Autodesk Inventor part; units mm, degrees
ref_plane "YZ Plane" through (0, 0, 0) normal (1, 0, 0) x (0, 1, 0)
ref_plane "XZ Plane" through (0, 0, 0) normal (0, 1, 0) x (-1, 0, 0)
ref_plane "XY Plane" through (0, 0, 0) normal (0, 0, 1) x (1, 0, 0)
sketch "Sketch1" plane through (0, 0, 0) normal (0, 1, 0) x (-1, 0, 0)
  line L0 (52.5, 30) -> (-52.5, 30)
  line L1 (-52.5, 30) -> (-52.5, -30)
  line L2 (-52.5, -30) -> (52.5, -30)
  line L3 (52.5, -30) -> (52.5, 30)
  line L4 (52.5, 0) -> (-52.5, 0) construction
  circle A0 centre (-42.5, 0) radius 1.5
  circle A1 centre (-0.5, 0) radius 1.5
  line L5 (-47.5, 25) -> (47.5, 25) construction
  line L6 (47.5, 25) -> (47.5, -25) construction
  line L7 (47.5, -25) -> (-47.5, -25) construction
  line L8 (-47.5, -25) -> (-47.5, 25) construction
  circle A2 centre (47.5, 25) radius 1.5
  circle A3 centre (47.5, -25) radius 1.5
  circle A4 centre (-47.5, 25) radius 1.5
  circle A5 centre (-47.5, -25) radius 1.5
  line L9 (47.5, 0) -> (34.5096, -7.5)
  line L10 (34.5096, -7.5) -> (34.5096, 7.5)
  line L11 (34.5096, 7.5) -> (47.5, 0)
  circle A6 centre (9.5, -13) radius 1
  circle A7 centre (9.5, 13) radius 1
  line L12 (9.5, -30) -> (9.5, 30) construction
  point P0 (0, 0)
  point P1 (0, 0)
  point P2 (38.8397, 0)
  dimension "d0" = 105
  dimension "d1" = 60
  dimension "d2" = 3
  dimension "d3" = 3
  dimension "d4" = 42
  dimension "d5" = 5
  dimension "d6" = 3
  dimension "d7" = 3
  dimension "d8" = 3
  dimension "d9" = 3
  dimension "d10" = 15
  dimension "d11" = 10
  dimension "d17" = 2
  dimension "d18" = 2
  dimension "d19" = 26
  dimension "d20" = 10
extrude "Extrusion1" add sketch "Sketch1" along normal blind 3
chamfer "Chamfer1" distance 2 angle 45 3 edges at (-41.0048, 3, -3.75) (-41.0048, 3, 3.75) (-34.5096, 3, 0)
properties part number "Front back" material "Iron, Gray"
Check sheet for the modelled part. Datum: model origin and axes. Units: mm. A direction names the side the tool comes from. Round coordinates to 2 decimals unless told otherwise and drop trailing zeros. Write each loop counter-clockwise with the first axis right and the second up, starting at its lowest first coordinate (ties: lowest second). Pieces come first, ordered by that corner, then holes. Notation, with made-up numbers: (20.25, 57.25) -> (63.25, 57.25) arc R20 cw to (63.25, 74.25) -> close; hole circle Ø3 at (-39.5, -8.5). An arc over 180 degrees is marked (long way). One line per question, with ' | ' between items. Start each with the question number.
1. Sectioned sample at A-A, the plane x = 47.5. Record the cut outline in (y, z), then the cut area to 3 significant figures.
2. Sectioned sample at B-B, the plane z = 13. Record the cut outline in (x, y).
3. Depth check by flat-ended pin: pin 1 (4 mm diameter, centred on x = -47.5, z = -25, fed in from -Y). Enter the tip coordinate at first touch or a pass-through.
4. Scan lines: line 1 along Z through (x, y) = (47.5, 1.3); line 2 along X through (y, z) = (1.25, 24.5); line 3 along Z through (x, y) = (-47.5, 1.5). Record each from-to range of solid material in increasing order. Write a range as from..to.
5. Set-up check for faces 5 (the face through (52.5, 1, 0)), 6 (the face through (-41.38, 2.01, -4.7)), 7 (the face through (-40.914, 0.493, 3.803)): record each of +Z, -Z, +X, -X, +Y, -Y from which the full face is reachable in a straight line by a thin tool's end or side.
6. Release check for a two-part mould opening along X. For faces 1 (the face through (44, 1, 0)), 2 (the face through (-52.5, 1, 0)), 3 (the face through (-46.39, 1.48, 23.99)), 4 (the face through (-1, 1, 30)) record: +X half, -X half, draft (parallel to the pull), parting line (faces both ways), or undercut.
7. Sectioned sample at C-C, the plane y = 2.45. Count the separate pieces of the cut face and the enclosed holes in it, then the cut area to 3 significant figures.
Taken from the geometry:
1) outline: (0, -30) -> (3, -30) -> (3, -26.5) -> (0, -26.5) -> close; (0, -23.5) -> (3, -23.5) -> (3, 23.5) -> (0, 23.5) -> close; (0, 26.5) -> (3, 26.5) -> (3, 30) -> (0, 30) -> close | area: 162 mm^2
2) outline: (-52.5, 0) -> (-10.5, 0) -> (-10.5, 3) -> (-52.5, 3) -> close; (-8.5, 0) -> (52.5, 0) -> (52.5, 3) -> (-8.5, 3) -> close
3) pin 1: stops at y = 0
4) line 1: z = -30..-26.5, -23.5..23.5, 26.5..30 | line 2: x = -52.5..-48.91, -46.09..46.09, 48.91..52.5 | line 3: z = -30..-26.5, -23.5..-0.58, 0.58..23.5, 26.5..30
5) face 5: +Z, -Z, +X, +Y, -Y | face 6: +Y | face 7: +Y, -Y
6) face 1: undercut | face 2: -X half | face 3: undercut | face 4: draft
7) separate pieces: 1 | enclosed holes: 9 | area: 6,080 mm^2
